Autodesk Inventor part; units mm, degrees
ref_plane "YZ Plane" through (0, 0, 0) normal (1, 0, 0) x (0, 1, 0)
ref_plane "XZ Plane" through (0, 0, 0) normal (0, 1, 0) x (-1, 0, 0)
ref_plane "XY Plane" through (0, 0, 0) normal (0, 0, 1) x (1, 0, 0)
sketch "Sketch1" plane through (0, 0, 0) normal (0, 0, 1) x (1, 0, 0)
  circle A0 centre (0, 0) radius 6.604
  arc A1 (0, 9.525) -> (0, -9.525) centre (0, 0) ccw
  line L0 (0, 9.525) -> (50.8, 9.525)
  line L1 (0, -9.525) -> (50.8, -9.525)
  arc A2 (50.8, -9.525) -> (50.8, 9.525) centre (50.8, 0) ccw
  dimension "d0" = 13.208
  dimension "d1" = 19.05
  dimension "d2" = 50.8
  dimension "d3" = 50.8
  dimension "d4" = 19.05
extrude "Extrusion1" add sketch "Sketch1" along normal blind 17.78
sketch "Sketch2" plane through (0, 0, 0) normal (0, 1, 0) x (-1, 0, 0)
  line L0 (9.525, 17.78) -> (0, 17.78)
  line L1 (9.525, 17.78) -> (9.525, 0)
  line L2 (9.525, 0) -> (9.525, 17.78)
  line L3 (0, 0) -> (0, 17.78)
  line L4 (9.525, 8.89) -> (0, 8.89)
  line L5 (0, 8.89) -> (0, 6.35)
  line L6 (0, 6.35) -> (9.525, 6.35)
  line L7 (9.525, 6.35) -> (9.525, 8.89)
  line L8 (9.525, 8.89) -> (0, 8.89)
  line L9 (0, 8.89) -> (0, 11.43)
  line L10 (0, 11.43) -> (9.525, 11.43)
  line L11 (9.525, 11.43) -> (9.525, 8.89)
  line L12 (0, 6.35) -> (-10.1637, 6.35)
  line L13 (-10.1637, 6.35) -> (-10.1637, 11.43)
  line L14 (-10.1637, 11.43) -> (0, 11.43)
  line L15 (0, 11.43) -> (0, 6.35)
  line L16 (9.525, 11.43) -> (-9.525, 11.43)
  line L17 (-9.525, 11.43) -> (-9.525, 6.35)
  line L18 (-9.525, 6.35) -> (9.525, 6.35)
  line L19 (9.525, 6.35) -> (9.525, 11.43)
  dimension "d8" = 2.54
  dimension "d9" = 2.54
  dimension "d10" = 19.05
extrude "Extrusion2" cut sketch "Sketch2" along normal mid plane 25.7175 contours L1 L4 L3 L10 | L3 L12 L17 L14 | L1 L6 L3 L4
sketch "Sketch3" plane through (0, 0, 0) normal (0, 1, 0) x (-1, 0, 0)
  line L0 (-50.8, 0) -> (-50.8, 17.78)
  circle A0 centre (-50.8, 8.89) radius 6.604
  point P0 (0, 0)
  dimension "d13" = 13.208
extrude "Extrusion3" cut sketch "Sketch3" along normal mid plane 25.7175
properties part number "toplegV2"
Read the model definition and answer for the solid it produces. Units are mm, in the model's axes. A direction names the side the tool comes from. Round coordinates to 2 decimals unless told otherwise and drop trailing zeros. Write each loop counter-clockwise with the first axis right and the second up, starting at its lowest first coordinate (ties: lowest second). Pieces come first, ordered by that corner, then holes. Notation, with made-up numbers: (-38.75, -36) - (-31.75, -36) arc R26 ccw to (-31.75, 3) - close; hole circle Ø6 at (62, 78.5). An arc over 180 degrees is marked (long way). Use a Markdown table: item, result.
(1) The part is cut by section D-D (x = 55). Write down the section's boundary in (y, z), then the cut area to 3 significant figures.
Reported:
| item | result |
|---|---|
| outline | (-8.55, 0) - (8.55, 0) - (8.55, 3.79) - (-8.55, 3.79) - close; (-8.55, 13.99) - (8.55, 13.99) - (8.55, 17.78) - (-8.55, 17.78) - close |
| area | 130 mm2 |
(2) Straight lines are drawn through the part: line 1 along X through (y, z) = (0, 16.25) (3 decimals); line 2 along Y through (x, z) = (0, 16) (3 decimals); line 3 along Z through (x, y) = (50.8, -3). For each, find the intervals that lie inside material, in ascending order. Write a range as [from, to].
Reported:
| item | result |
|---|---|
| line 1 | [-9.525, -6.604], [6.604, 60.325] |
| line 2 | [-9.525, -6.604], [6.604, 9.525] |
| line 3 | [0, 2.29], [15.49, 17.78] |
(3) The part is cut by section B-B (z = 12.75). Write down the section's boundary in (x, y) (3 decimals).
Reported:
| item | result |
|---|---|
| outline | (0, -9.525) - (45.442, -9.525) - (45.442, 9.525) - (0, 9.525) arc R9.525 ccw to start; (56.158, -7.875) arc R9.525 ccw to (56.158, 7.875) - close; hole circle Ø13.208 at (0, 0) |
(4) Which of the six approach directions +Z, -Z, +X, -X, +Y, -Y give full straight-line access (tool end or side, diameter ignored) to faces 1 (the flat face through (25, 0, 17.78)), 2 (the flat face through (9.525, 0, 9))?
Reported:
| item | result |
|---|---|
| face 1 | +Z, +X, -X, +Y, -Y |
| face 2 | -X, +Y, -Y |
(5) Each of these flat-tipped pins is pushed along its axis until it touches: pin 1 Ø1 at (y, z) = (2, 10.5) entering from +X; pin 2 Ø6 at (y, z) = (-1.5, 11.5) entering from +X (3 decimals); pin 3 Ø5 at (y, z) = (5, 13) entering from +X; pin 4 Ø1.5 at (y, z) = (-0.5, 8) entering from -X (3 decimals). Where does it stop, or does it pass through?
Reported:
| item | result |
|---|---|
| pin 1 | x = 60.21 |
| pin 2 | x = 60.325 |
| pin 3 | x = 59.99 |
| pin 4 | x = 9.525 |
(6) The part is cut by section C-C (x = -1.5). Write down the section's boundary in (y, z), then the cut area to 3 significant figures.
Reported:
| item | result |
|---|---|
| outline | (-9.41, 0) - (-6.43, 0) - (-6.43, 6.35) - (-9.41, 6.35) - close; (-9.41, 11.43) - (-6.43, 11.43) - (-6.43, 17.78) - (-9.41, 17.78) - close; (6.43, 0) - (9.41, 0) - (9.41, 6.35) - (6.43, 6.35) - close; (6.43, 11.43) - (9.41, 11.43) - (9.41, 17.78) - (6.43, 17.78) - close |
| area | 75.6 mm2 |
(7) The part is cut by section A-A (y = 4). Write down the section's boundary in (x, z) (3 decimals), then the cut area to 3 significant figures.
Reported:
| item | result |
|---|---|
| outline | (-8.644, 0) - (-5.255, 0) - (-5.255, 6.35) - (-8.644, 6.35) - close; (-8.644, 11.43) - (-5.255, 11.43) - (-5.255, 17.78) - (-8.644, 17.78) - close; (5.255, 0) - (59.444, 0) - (59.444, 17.78) - (5.255, 17.78) - (5.255, 11.43) - (9.525, 11.43) - (9.525, 6.35) - (5.255, 6.35) - close; hole circle Ø13.208 at (50.8, 8.89) |
| area | 848 mm2 |
(8) The mould has two halves that part along Z. Classify faces 3 (the cylindrical face through (6.1, 2.53, 3.13)), 4 (the flat face through (25, 0, 0)), 5 (the flat face through (6.5, -2.3, 6.35)): released by +Z, released by -Z, zero draft, split by the parting line, or undercut.
Reported:
| item | result |
|---|---|
| face 3 | zero draft |
| face 4 | released by -Z |
| face 5 | undercut |
